Drawing for the job (mm, zero at the part's lowest x, y, z). A direction names the side the tool comes from. Give positions to 0.01 mm unless a question says otherwise; leave off trailing zeros. Order: outer loops, then holes, each group sorted by start corner. A loop starts at its lowest first (then second) coordinate and runs counter-clockwise, first axis right, second up. Notation, with made-up numbers: (-18.75, 5.25) - (-12.75, 5.25) arc R7 cw to (-12.75, 12.25) - close; hole circle Ø2 at (79, 13). An arc over 180 degrees is marked (long way). One line per item, written item: value.
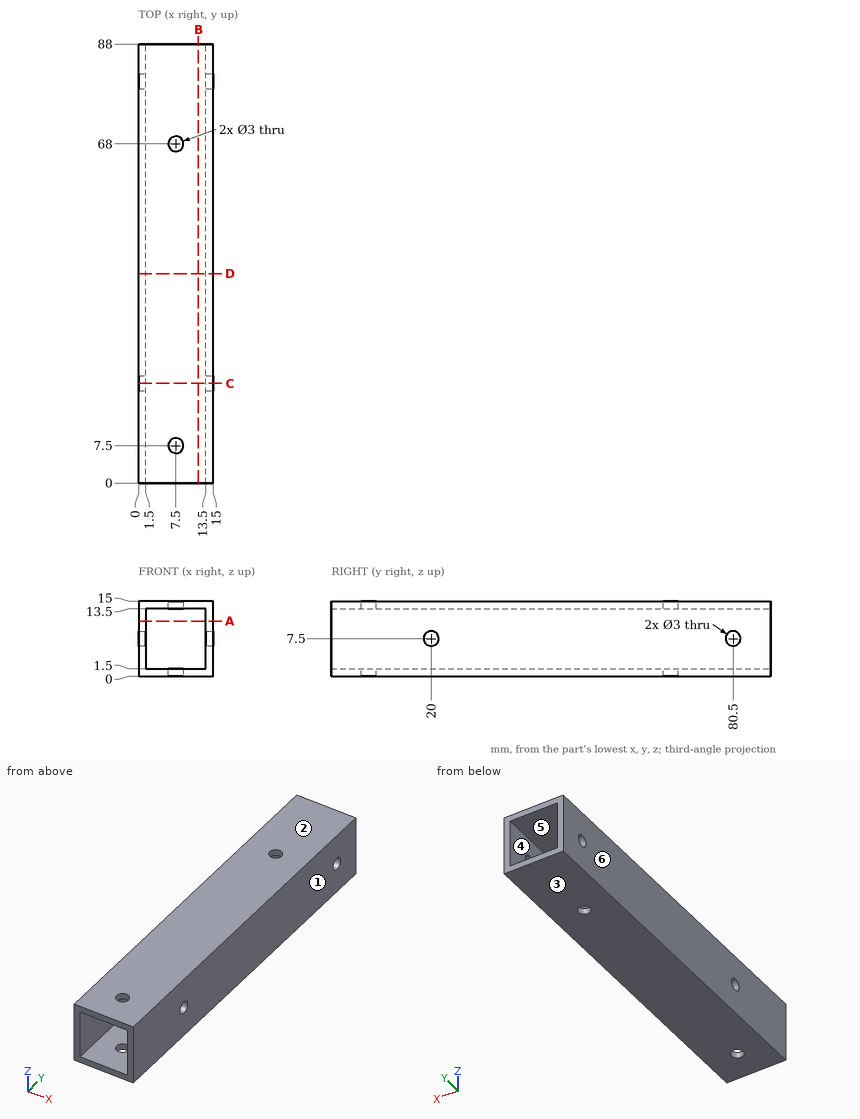
1) Cut at B-B, the plane x = 12. Give the cut face in (y, z), then the cut area to 3 significant figures.
Outcome:
outline: (0, 0) - (88, 0) - (88, 1.5) - (0, 1.5) - close; (0, 13.5) - (88, 13.5) - (88, 15) - (0, 15) - close
area: 264 mm^2
2) Which spindle directions (+Z, -Z, +X, -X, +Y, -Y) get a long thin tool onto all of the face, cutting with end or side? Do the marked faces 5 and 6. Say none if no direction does.
Outcome:
face 5: +Y, -Y
face 6: +Z, -Z, -X, +Y, -Y
3) Mould opens along Z. For the marked faces 1, 2, 3 and 4 say: released by +Z, released by -Z, zero draft, split by the parting line, or undercut.
Outcome:
face 1: zero draft
face 2: released by +Z
face 3: released by -Z
face 4: undercut
4) Cut at C-C, the plane y = 20. Give the cut face in (x, z).
Outcome:
outline: (0, 0) - (15, 0) - (15, 6) - (13.5, 6) - (13.5, 1.5) - (1.5, 1.5) - (1.5, 6) - (0, 6) - close; (0, 9) - (1.5, 9) - (1.5, 13.5) - (13.5, 13.5) - (13.5, 9) - (15, 9) - (15, 15) - (0, 15) - close
5) Drill centre lines: line 1 along Y through (x, z) = (0.75, 7.5); line 2 along Z through (x, y) = (12, 75.5). Where is each one in solid material? Low to high. Write a range as from..to.
Outcome:
line 1: y = 0..18.5, 21.5..79, 82..88
line 2: z = 0..1.5, 13.5..15
6) Cut at D-D, the plane y = 42. Give the cut face in (x, z).
Outcome:
outline: (0, 0) - (15, 0) - (15, 15) - (0, 15) - close; hole (1.5, 1.5) - (13.5, 1.5) - (13.5, 13.5) - (1.5, 13.5) - close
7) Cut at A-A, the plane z = 11. Give the cut face in (x, y), then the cut area to 3 significant figures.
Outcome:
outline: (0, 0) - (1.5, 0) - (1.5, 88) - (0, 88) - close; (13.5, 0) - (15, 0) - (15, 88) - (13.5, 88) - close
area: 264 mm^2
